The model under review builds one solid part; all positions refer to its coordinate system, in mm. Round coordinates to 2 decimals unless told otherwise and drop trailing zeros. Loops run counter-clockwise (first coordinate to the right, second up) from the corner with the lowest first, then second, coordinate; pieces in that order, holes last. Notation, with made-up numbers: M 71.5,-5 L 94.5,-5 A19 cw 94.5,22 Z; hole C 84,81.5 d6. An arc over 180 degrees is marked long. Answer as a JSON object with one key per item and string values. Group by question number.
Item 1: To check wall thickness, follow line 1 (X direction, y = 0.95, z = -0.25); line 2 (Z direction, x = 134.5, y = 1.75); line 3 (X direction, y = 0.65, z = 5.5). State the ranges of each line that lie inside material, in increasing order.
Item 2: Consider section D-D (x = -4.5). Give the boundary of the cut face in (y, z).
Item 3: Consider section B-B (y = 4). Give the boundary of the cut face in (x, z), and give its area (3 significant figures).
Item 4: Consider section A-A (z = -4.75). Give the boundary of the cut face in (x, y), and give its area (3 significant figures).
Item 5: Consider section C-C (x = 59). Give the boundary of the cut face in (y, z).
Item 6: Insertion check: P1, Ø1.5, axis at y = 1.5, z = -18.5, coming from the +X side; P2, Ø4, axis at x = 118.25, z = 3.33, coming from the -Y side; P3, Ø2.5, axis at y = 3, z = -18, coming from the -X side; P4, Ø2.5, axis at x = 137, y = 1.5, coming from the -Z side. Each pin has a flat end and moves straight along its axis. Give the tip position at first contact, or say it passes through.
```python
from build123d import *

# Parameters (mm, degrees)
SKETCH1_W            = 208
SKETCH1_H            = 25
BOSS_EXTRUDE1_DEPTH  = 5
SURUCU_BOSLUGU_DEPTH = 6
SKETCH7_R            = 2.1
KASA_BAGLANTI_DEPTH  = 6
SKETCH8_W            = 15
SKETCH8_H            = 3
YAN_BAGLANTI_DEPTH   = 5


with BuildPart() as part:
    # Sketch1 → Boss-Extrude1 (new body)
    with BuildSketch(Plane(origin=(0, 0, 0), x_dir=(1, 0, 0), z_dir=(0, 1, 0))):
        with Locations((44.254700849, 4.167980547)):
            Rectangle(SKETCH1_W, SKETCH1_H)
    extrude(amount=BOSS_EXTRUDE1_DEPTH)

    # Sketch6 → Surucu Boslugu (cut, through all)
    with BuildSketch(Plane(origin=(0, 0, 0), x_dir=(-1, 0, 0), z_dir=(0, -1, 0))):
        with BuildLine():
            Line((-72.254700849, -8.332019453), (-7.254700849, -8.332019453))
            ThreePointArc((-7.254700849, -8.332019453), (-10.790234755, -6.867553359), (-12.254700849, -3.332019453))
            Line((-12.254700849, -3.332019453), (-12.254700849, 6.667980547))
            ThreePointArc((-12.254700849, 6.667980547), (-13.719166943, 10.203514453), (-17.254700849, 11.667980547))
            Line((-17.254700849, 11.667980547), (-62.254700849, 11.667980547))
            ThreePointArc((-62.254700849, 11.667980547), (-65.790234755, 10.203514453), (-67.254700849, 6.667980547))
            Line((-67.254700849, 6.667980547), (-67.254700849, -3.332019453))
            ThreePointArc((-67.254700849, -3.332019453), (-68.719166943, -6.867553359), (-72.254700849, -8.332019453))
        make_face()
    extrude(amount=-SURUCU_BOSLUGU_DEPTH, mode=Mode.SUBTRACT)

    # Sketch7 → Kasa Baglanti (cut, through all)
    with BuildSketch(Plane.XZ):
        with Locations((-29.745299151, 3.332019453)):
            Circle(SKETCH7_R)
        with Locations((118.254700849, 3.332019453)):
            Circle(SKETCH7_R)
    extrude(amount=-KASA_BAGLANTI_DEPTH, mode=Mode.SUBTRACT)

    # Sketch8 → Yan Baglanti (add, through all)
    with BuildSketch(Plane.XZ):
        with Locations((124.254700849, -18.167980547)):
            Rectangle(SKETCH8_W, SKETCH8_H)
        with Locations((44.254700849, -18.167980547)):
            Rectangle(SKETCH8_W, SKETCH8_H)
        with Locations((-35.745299151, -18.167980547)):
            Rectangle(SKETCH8_W, SKETCH8_H)
    extrude(amount=-YAN_BAGLANTI_DEPTH)


solid = part.part
```
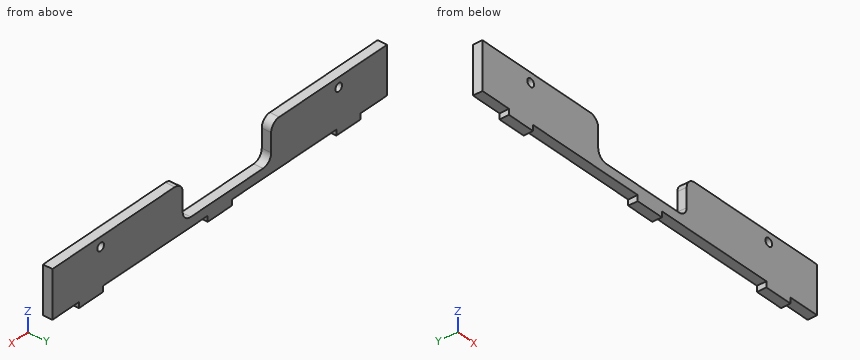
Geometry results:
{
 "1": {"line 1": "x = -59.75 to 12.25, 67.25 to 148.25", "line 2": "z = -16.67 to 8.33", "line 3": "x = -59.75 to 11.76, 67.75 to 148.25"},
 "2": {"outline": "M 0,-16.67 L 5,-16.67 L 5,8.33 L 0,8.33 Z"},
 "3": {"outline": "M -59.75,-16.67 L -43.25,-16.67 L -43.25,-19.67 L -28.25,-19.67 L -28.25,-16.67 L 36.75,-16.67 L 36.75,-19.67 L 51.75,-19.67 L 51.75,-16.67 L 116.75,-16.67 L 116.75,-19.67 L 131.75,-19.67 L 131.75,-16.67 L 148.25,-16.67 L 148.25,8.33 L 72.25,8.33 A5 ccw 67.25,3.33 L 67.25,-6.67 A5 cw 62.25,-11.67 L 17.25,-11.67 A5 cw 12.25,-6.67 L 12.25,3.33 A5 ccw 7.25,8.33 L -59.75,8.33 Z; hole C -29.75,3.33 d4.2; hole C 118.25,3.33 d4.2", "area": "4,210 mm^2"},
 "4": {"outline": "M -59.75,0 L 12.25,0 L 12.25,5 L -59.75,5 Z; M 67.25,0 L 148.25,0 L 148.25,5 L 67.25,5 Z", "area": "765 mm^2"},
 "5": {"outline": "M 0,-16.67 L 5,-16.67 L 5,-11.67 L 0,-11.67 Z"},
 "6": {"P1": "stops at x = 131.75", "P2": "passes through", "P3": "stops at x = -43.25", "P4": "stops at z = -16.67"}
}
